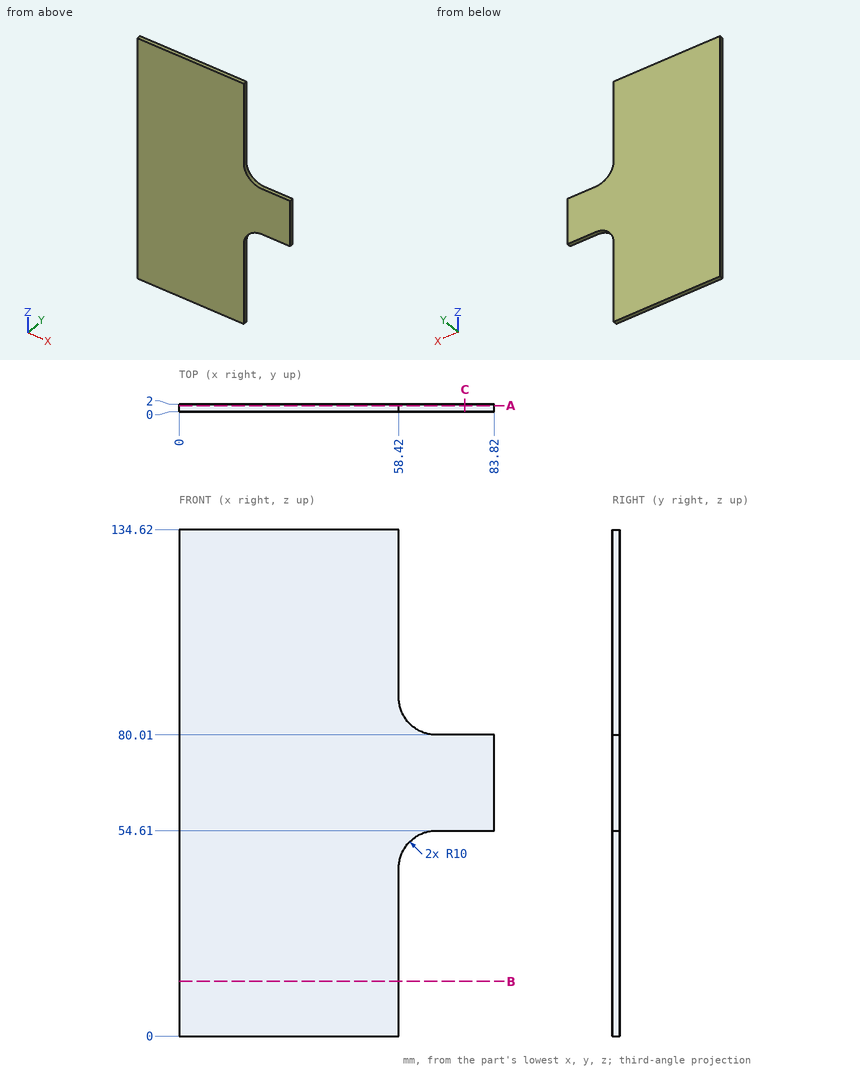
Input: dimensioned drawing with shaded views. Units: mm. Origin: part minimum x, y, z. Give positions to 0.01 mm unless a question says otherwise; leave off trailing zeros. Write each loop counter-clockwise with the first axis right and the second up, starting at its lowest first coordinate (ties: lowest second). Pieces come first, ordered by that corner, then holes. Notation, with made-up numbers: M 60.5,-30 L 65.5,-30 A10 cw 65.5,-14 Z; hole C 17,80.5 d1. An arc over 180 degrees is marked long. Return JSON: item names as keys, results as strings. Group by question number.
1) Cut plane B-B, the plane z = 14.5. Output: boundary loops of the cut face in (x, y), plus the area to 3 significant figures.
2) Cut plane C-C, the plane x = 76. Output: boundary loops of the cut face in (y, z).
3) Material intervals for line 1 along X through (y, z) = (1.55, 27); line 2 along Z through (x, y) = (68.5, 1.1); line 3 along X through (y, z) = (1.4, 82.5), sorted ascending. Write a range as [from, to].
4) Pin query (flat end, axial travel): P1, Ø0.6, axis at x = 72.5, y = 1, coming from the -Z side. Return the tip coordinate at first contact, or that it passes through.
5) Cut plane A-A, the plane y = 1.6. Output: boundary loops of the cut face in (x, z), plus the area to 3 significant figures.
Recorded:
{
 "1": {"outline": "M 0,0 L 58.42,0 L 58.42,2 L 0,2 Z", "area": "117 mm²"},
 "2": {"outline": "M 0,54.61 L 2,54.61 L 2,80.01 L 0,80.01 Z"},
 "3": {"line 1": "x = [0, 58.42]", "line 2": "z = [54.61, 80.01]", "line 3": "x = [0, 61.82]"},
 "4": {"P1": "stops at z = 54.61"},
 "5": {"outline": "M 0,0 L 58.42,0 L 58.42,44.61 A10 cw 68.42,54.61 L 83.82,54.61 L 83.82,80.01 L 68.42,80.01 A10 cw 58.42,90.01 L 58.42,134.62 L 0,134.62 Z", "area": "8,550 mm²"}
}
